The model under review builds one solid part; all positions refer to its coordinate system, in mm. Face numbers are marked on the shaded views. A direction names the side the tool comes from. Round coordinates to 2 decimals unless told otherwise and drop trailing zeros. Order: outer loops, then holes, each group sorted by start corner. A loop starts at its lowest first (then second) coordinate and runs counter-clockwise, first axis right, second up.
1) Consider section A-A (y = 166.5). Give the boundary of the cut face in (x, z).
2) Consider section B-B (z = 150). Give the boundary of the cut face in (x, y).
3) To check wall thickness, follow L1, parallel to Y at x = 14, z = 154; L2, parallel to Z at x = 19.05, y = 176; L3, parallel to Z at x = -19.05, y = 175. State the ranges of each line that lie inside material, in increasing order.
4) Machinability: for the marked faces 1 and 2, which of the approach directions +Z, -Z, +X, -X, +Y, -Y give a long, thin tool a straight path to every point of the face, cutting with its end or side? Answer none if there is none.
5) Clearance check with flat-ended pins moving along their axes: P1, Ø2, axis at x = -26, z = 147.5, coming from the -Y side; P2, Ø2, axis at x = 7, y = 161, coming from the -Z side; P3, Ø3, axis at y = 157.5, z = 174.5, coming from the +X side. State where each tip first meets the part, or that it passes through.
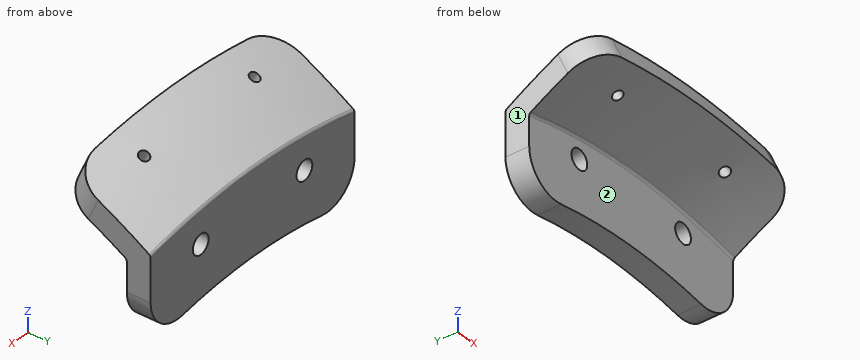
from build123d import *

# Parameters (mm, degrees)
REVOLVE1_ANGLE     = 30.000000000000068
SKETCH5_OUTSIDE_W  = 117.778
SKETCH5_OUTSIDE_H  = 65.886
CUT_EXTRUDE2_DEPTH = 260.76149135356775
FILLET1_R          = 10
FILLET2_R          = 1
SKETCH6_R          = 2.9000000000000363
CUT_EXTRUDE3_DEPTH = 189.07070419365607


with BuildPart() as part:
    # Sketch1 → Revolve1 (revolve, symmetric)
    with BuildSketch(Plane(origin=(0, 0, 0), x_dir=(0, 0, -1), z_dir=(1, 0, 0))) as revolve1_sk:
        with BuildLine():
            Line((-182.35774731109075, 155.06255495822683), (-175.97602387063264, 152.18616730537))
            ThreePointArc((-175.97602387063264, 152.18616730537), (-171.12326361620543, 162.17531665611477), (-165.70405663890074, 171.86884968466347))
            Line((-165.70405663890074, 171.86884968466347), (-144.78715490957802, 171.8688496846635))
            Line((-144.78715490957802, 171.8688496846635), (-144.78715490957802, 178.86884968466353))
            Line((-144.78715490957802, 178.86884968466353), (-169.62958875117425, 178.8688496846635))
            ThreePointArc((-169.62958875117425, 178.8688496846635), (-176.3957372053048, 167.18067068421345), (-182.35774731109075, 155.06255495822683))
        make_face()
    revolve(axis=Axis((0, 0, 0), (0, 1, 0)), revolution_arc=REVOLVE1_ANGLE / 2)
    revolve(revolve1_sk.sketch, axis=Axis((0, 0, 0), (0, -1, 0)), revolution_arc=REVOLVE1_ANGLE / 2)

    # Sketch4 → Cut-Revolve1 (revolve, cut)
    with BuildSketch(Plane(origin=(0, 57.85077924674397, -29.47644429930001), x_dir=(0, 0.4539904997395446, 0.891006524188369), z_dir=(0, -0.891006524188369, 0.4539904997395446)), mode=Mode.PRIVATE) as cut_revolve1_sk:
        Polygon((200.3216852155454, 19.031606271083962), (239.0176946479082, 22.417068420107935), (239.1484282620297, 20.922776372970326), (200.4524188296669, 17.53731422394635), align=None)
    cut_revolve1 = revolve(cut_revolve1_sk.sketch.rotate(Axis((-17.53731422394635, 148.85427304522494, 149.12796866727265), (-0.08715574274765833, 0.4522629288245563, 0.8876159753616077)), 8.229125289), axis=Axis((-17.53731422394635, 148.85427304522494, 149.12796866727265), (-0.08715574274765833, 0.4522629288245563, 0.8876159753616077)), mode=Mode.SUBTRACT)

    # Mirror1: Cut-Revolve1 across plane
    add(cut_revolve1.mirror(Plane(origin=(0, 0, 0), x_dir=(0, 0, 1), z_dir=(1, 0, 0))), mode=Mode.SUBTRACT)

    # Sketch5 outside → Cut-Extrude2 (cut, through all)
    with BuildSketch(Plane(origin=(0, 0, 0), x_dir=(1, 0, 0), z_dir=(0, 1, 0))):
        with Locations((0, -161.106)):
            Rectangle(SKETCH5_OUTSIDE_W, SKETCH5_OUTSIDE_H)
        Polygon((37.473673176807814, -139.85365224207746), (-37.473673176807814, -139.85365224207746), (-37.47367317680781, -182.35774731109072), (37.47367317680782, -182.35774731109072), align=None, mode=Mode.SUBTRACT)
    extrude(amount=CUT_EXTRUDE2_DEPTH, mode=Mode.SUBTRACT)

    # Fillet1
    fillet1_edges = [part.edges().sort_by_distance(p)[0] for p in [
        (37.47367317680782, 175.36884968466353, 139.85365224207746),
        (37.47367317680782, 153.6238703887916, 175.2030438132355),
        (-37.47367317680781, 153.6238703887916, 175.20304381323552),
        (-37.47367317680782, 175.36884968466353, 139.85365224207746),
    ]]
    fillet(fillet1_edges, radius=FILLET1_R)

    # Fillet2
    fillet2_edges = [part.edges().sort_by_distance(p)[0] for p in [
        (2.132e-14, 178.86884968466353, 169.62958875117428),
        (1.421e-14, 171.86884968466347, 165.7040566389007),
    ]]
    fillet(fillet2_edges, radius=FILLET2_R)

    # Sketch6 → Cut-Extrude3 (cut, through all)
    with BuildSketch(Plane(origin=(0, 178.8688496846635, 0), x_dir=(1, 0, 0), z_dir=(0, 1, 0))):
        with Locations(Location((19.049999999999898, -158.67424557151682, 0), (0, 0, 270))):
            Circle(SKETCH6_R)
        with Locations(Location((-19.050000000000104, -158.67424557151682, 0), (0, 0, 270))):
            Circle(SKETCH6_R)
    extrude(amount=-CUT_EXTRUDE3_DEPTH, mode=Mode.SUBTRACT)


solid = part.part
Answer below:
1. outline: (-37.47, 164.58) arc R168.8 cw to (37.47, 164.58) - (37.47, 172.74) arc R176.76 ccw to (-37.47, 172.74) - close
2. outline: (-37.2, 171.87) - (37.2, 171.87) - (37.2, 178.87) - (-37.2, 178.87) - close
3. L1: y = 171.87 to 178.87
3. L2: z = 143.53 to 155.77, 161.57 to 170.33
3. L3: z = 143.53 to 155.77, 161.57 to 170.93
4. face 1: +Z, -Z, -X, +Y, -Y
4. face 2: -Z, -Y
5. P1: stops at y = 171.87
5. P2: stops at z = 171.07
5. P3: stops at x = 36.66
